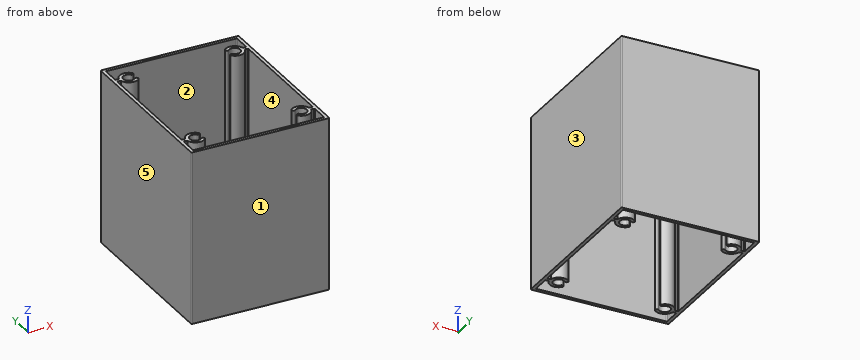
```python
from build123d import *

# Parameters (mm, degrees)
F1_DEPTH = 100


# Not quite as in the source:
# - ends of sketch curves that miss each other by under 0.0002 mm in the source are joined


with BuildPart() as f1:
    # F0 (on Top) → F1 (new body)
    with BuildSketch(Plane.XY):
        with BuildLine():
            Line((40, -49.5), (40, 49.5))
            ThreePointArc((40, 49.5), (39.8535533906, 49.8535533906), (39.5, 50))
            Line((39.5, 50), (-39.5, 50))
            ThreePointArc((-39.5, 50), (-39.8535533906, 49.8535533906), (-40, 49.5))
            Line((-40, 49.5), (-40, -49.5))
            ThreePointArc((-40, -49.5), (-39.8535533906, -49.8535533906), (-39.5, -50))
            Line((-39.5, -50), (39.5, -50))
            ThreePointArc((39.5, -50), (39.8535533906, -49.8535533906), (40, -49.5))
        make_face()
        with BuildLine():
            ThreePointArc((37.5, 48), (37.8535533906, 47.8535533906), (38, 47.5))
            Line((38, 47.5), (38, 38))
            ThreePointArc((38, 38), (37.8535533906, 37.6464466094), (37.5, 37.5))
            Line((37.5, 37.5), (36.300901, 37.5))
            ThreePointArc((36.300901, 37.5), (35.9969413236, 37.6030006107), (35.8182137763, 37.8695659396))
            ThreePointArc((35.8182137763, 37.8695659396), (32.0417405862, 41.5886055318), (26.9486644214, 40.1210975986))
            ThreePointArc((26.9486644214, 40.1210975986), (26.6829406294, 39.2888133915), (27.1727282582, 38.5653394472))
            ThreePointArc((27.1727282582, 38.5653394472), (27.8152796085, 38.4415776294), (28.396791896, 38.7416320991))
            ThreePointArc((28.396791896, 38.7416320991), (34, 36.499999638), (28.3967917139, 34.2583687274))
            ThreePointArc((28.3967917139, 34.2583687274), (27.815279361, 34.5584234062), (27.1727278252, 34.4346613028))
            ThreePointArc((27.1727278252, 34.4346613028), (26.6829405938, 33.711187361), (26.948664104, 32.8789030991))
            ThreePointArc((26.948664104, 32.8789030991), (32.0417407031, 31.4113944979), (35.8182138677, 35.1304350358))
            ThreePointArc((35.8182138677, 35.1304350358), (35.9969417068, 35.3969996827), (36.300901, 35.5))
            Line((36.300901, 35.5), (37.5, 35.5))
            ThreePointArc((37.5, 35.5), (37.8535533906, 35.3535533906), (38, 35))
            Line((38, 35), (38, -35.000003))
            ThreePointArc((38, -35.000003), (37.8535533906, -35.3535563906), (37.5, -35.500003))
            Line((37.5, -35.500003), (36.300901, -35.500003))
            ThreePointArc((36.300901, -35.500003), (35.9969417068, -35.3970026827), (35.8182140282, -35.1304379924))
            ThreePointArc((35.8182140282, -35.1304379924), (32.0417407032, -31.4113974979), (26.948663922, -32.8789059257))
            ThreePointArc((26.948663922, -32.8789059257), (26.6829405938, -33.711190361), (27.1727278252, -34.4346643028))
            ThreePointArc((27.1727278252, -34.4346643028), (27.815279361, -34.5584264062), (28.396791896, -34.2583719009))
            ThreePointArc((28.396791896, -34.2583719009), (34, -36.500002638), (28.3967922133, -38.7416347968))
            ThreePointArc((28.3967922133, -38.7416347968), (27.8152796085, -38.4415806294), (27.1727282582, -38.5653424472))
            ThreePointArc((27.1727282582, -38.5653424472), (26.6829406294, -39.2888163915), (26.948664104, -40.1211009009))
            ThreePointArc((26.948664104, -40.1211009009), (32.0417405862, -41.5886085318), (35.8182136159, -37.8695688962))
            ThreePointArc((35.8182136159, -37.8695688962), (35.9969413236, -37.6030036107), (36.300901, -37.500003))
            Line((36.300901, -37.500003), (37.5, -37.500003))
            ThreePointArc((37.5, -37.500003), (37.8535533906, -37.6464496094), (38, -38.000003))
            Line((38, -38.000003), (38, -47.5))
            ThreePointArc((38, -47.5), (37.8535533906, -47.8535533906), (37.5, -48))
            Line((37.5, -48), (-37.5, -48))
            ThreePointArc((-37.5, -48), (-37.8535533906, -47.8535533906), (-38, -47.5))
            Line((-38, -47.5), (-38, -38.000003))
            ThreePointArc((-38, -38.000003), (-37.8535533906, -37.6464496094), (-37.5, -37.500003))
            Line((-37.5, -37.500003), (-36.300901, -37.500003))
            ThreePointArc((-36.300901, -37.500003), (-35.9969413236, -37.6030036107), (-35.8182137763, -37.8695689396))
            ThreePointArc((-35.8182137763, -37.8695689396), (-32.0417405862, -41.5886085318), (-26.9486644214, -40.1211005986))
            ThreePointArc((-26.9486644214, -40.1211005986), (-26.6829406294, -39.2888163915), (-27.1727282582, -38.5653424472))
            ThreePointArc((-27.1727282582, -38.5653424472), (-27.8152796085, -38.4415806294), (-28.396791896, -38.7416350991))
            ThreePointArc((-28.396791896, -38.7416350991), (-34, -36.500002638), (-28.3967917139, -34.2583717274))
            ThreePointArc((-28.3967917139, -34.2583717274), (-27.815279361, -34.5584264062), (-27.1727278252, -34.4346643028))
            ThreePointArc((-27.1727278252, -34.4346643028), (-26.6829405938, -33.711190361), (-26.948664104, -32.8789060991))
            ThreePointArc((-26.948664104, -32.8789060991), (-32.0417407032, -31.4113974979), (-35.8182138677, -35.1304380358))
            ThreePointArc((-35.8182138677, -35.1304380358), (-35.9969417068, -35.3970026827), (-36.300901, -35.500003))
            Line((-36.300901, -35.500003), (-37.5, -35.500003))
            ThreePointArc((-37.5, -35.500003), (-37.8535533906, -35.3535563906), (-38, -35.000003))
            Line((-38, -35.000003), (-38, 35))
            ThreePointArc((-38, 35), (-37.8535533906, 35.3535533906), (-37.5, 35.5))
            Line((-37.5, 35.5), (-36.300901, 35.5))
            ThreePointArc((-36.300901, 35.5), (-35.9969417068, 35.3969996827), (-35.8182140282, 35.1304349924))
            ThreePointArc((-35.8182140282, 35.1304349924), (-32.0417407031, 31.4113944979), (-26.948663922, 32.8789029257))
            ThreePointArc((-26.948663922, 32.8789029257), (-26.6829405938, 33.711187361), (-27.1727278252, 34.4346613028))
            ThreePointArc((-27.1727278252, 34.4346613028), (-27.815279361, 34.5584234062), (-28.396791896, 34.2583689009))
            ThreePointArc((-28.396791896, 34.2583689009), (-34, 36.499999638), (-28.3967922133, 38.7416317968))
            ThreePointArc((-28.3967922133, 38.7416317968), (-27.8152796085, 38.4415776294), (-27.1727282582, 38.5653394472))
            ThreePointArc((-27.1727282582, 38.5653394472), (-26.6829406294, 39.2888133915), (-26.948664104, 40.1210979009))
            ThreePointArc((-26.948664104, 40.1210979009), (-32.0417405862, 41.5886055318), (-35.8182136159, 37.8695658962))
            ThreePointArc((-35.8182136159, 37.8695658962), (-35.9969413236, 37.6030006107), (-36.300901, 37.5))
            Line((-36.300901, 37.5), (-37.5, 37.5))
            ThreePointArc((-37.5, 37.5), (-37.8535533906, 37.6464466094), (-38, 38))
            Line((-38, 38), (-38, 47.5))
            ThreePointArc((-38, 47.5), (-37.8535533906, 47.8535533906), (-37.5, 48))
            Line((-37.5, 48), (37.5, 48))
        make_face(mode=Mode.SUBTRACT)
    extrude(amount=-F1_DEPTH)


solid = f1.part
```
Can you work these out from the model? Positions are in its coordinate system, mm. Face numbers are marked on the shaded views. A direction names the side the tool comes from. Give positions to 0.01 mm unless a question says otherwise; leave off trailing zeros. Order: outer loops, then holes, each group sorted by start corner. A loop starts at its lowest first (then second) coordinate and runs counter-clockwise, first axis right, second up. Notation, with made-up numbers: M 57.5,-28.75 L 63.5,-28.75 A16 ccw 63.5,-12.75 Z; hole C 41.25,-9 d7. An arc over 180 degrees is marked long. Write item = value, one per line. Start each with the question number.
Q1. Suppose I cut it at C-C (x = -30.75). Write out the boundary of the cut face in (y, z).
Q2. For the marked faces 1 and 2, which set-ups out of +Z, -Z, +X, -X, +Y, -Y let a thin tool reach every point of the face, with its end or its side?
Q3. We'd pull the mould along X, two halves only. Please class the marked faces 3, 4 and 5: pulls with the +X half, pulls with the -X half, needs draft (parallel to the pull), parting line crosses it, or undercut.
Q4. I need wall thicknesses on probe 1 along Y at (x, z) = (-30.75, -19.5); probe 2 along X at (y, z) = (-25, -79); probe 3 along X at (y, z) = (39, -4.5). Which ranges of each line are inside material? Lowest first, please. Write a range as [from, to].
Q5. Will this pin go through, and if not, where does the flat tip stop? pin 1 Ø6 at (x, y) = (-30.75, -36.5) entering from +Z.
Q6. Suppose I cut it at A-A (x = 16.5). Write out the boundary of the cut face in (y, z).
Q7. Suppose I cut it at B-B (y = -11). Write out the boundary of the cut face in (x, z), plus the area to 3 significant figures.
Check result:
q1.outline = M -50,-100 L -48,-100 L -48,0 L -50,0 Z; M -41.75,-100 L -39.75,-100 L -39.75,0 L -41.75,0 Z; M -33.25,-100 L -31.25,-100 L -31.25,0 L -33.25,0 Z; M 31.25,-100 L 33.25,-100 L 33.25,0 L 31.25,0 Z; M 39.75,-100 L 41.75,-100 L 41.75,0 L 39.75,0 Z; M 48,-100 L 50,-100 L 50,0 L 48,0 Z
q2.face_1 = +Z, -Z, +X, -X, -Y
q2.face_2 = +Z, -Z
q3.face_3 = pulls with the +X half
q3.face_4 = undercut
q3.face_5 = pulls with the -X half
q4.probe_1 = [-50, -48], [-41.75, -39.75], [-33.25, -31.25], [31.25, 33.25], [39.75, 41.75], [48, 50]
q4.probe_2 = [-40, -38], [38, 40]
q4.probe_3 = [-40, -38], [-35.37, -32.83], [-28.67, -26.77], [26.77, 28.67], [32.83, 35.37], [38, 40]
q5.pin_1 = through
q6.outline = M -50,-100 L -48,-100 L -48,0 L -50,0 Z; M 48,-100 L 50,-100 L 50,0 L 48,0 Z
q7.outline = M -40,-100 L -38,-100 L -38,0 L -40,0 Z; M 38,-100 L 40,-100 L 40,0 L 38,0 Z
q7.area = 400 mm2
